Geometry: see drawing. Coordinates: mm, zero at the bounding-box minimum. A direction names the side the tool comes from. Round coordinates to 2 decimals unless told otherwise and drop trailing zeros. Write each loop counter-clockwise with the first axis right and the second up, starting at its lowest first coordinate (ties: lowest second). Pieces come first, ordered by that corner, then holes. Notation, with made-up numbers: M 66,32.5 L 105,32.5 A30 cw 105,56.5 Z; hole C 87.25,40 d7. An arc over 180 degrees is marked long. Use a Markdown table: item, result.
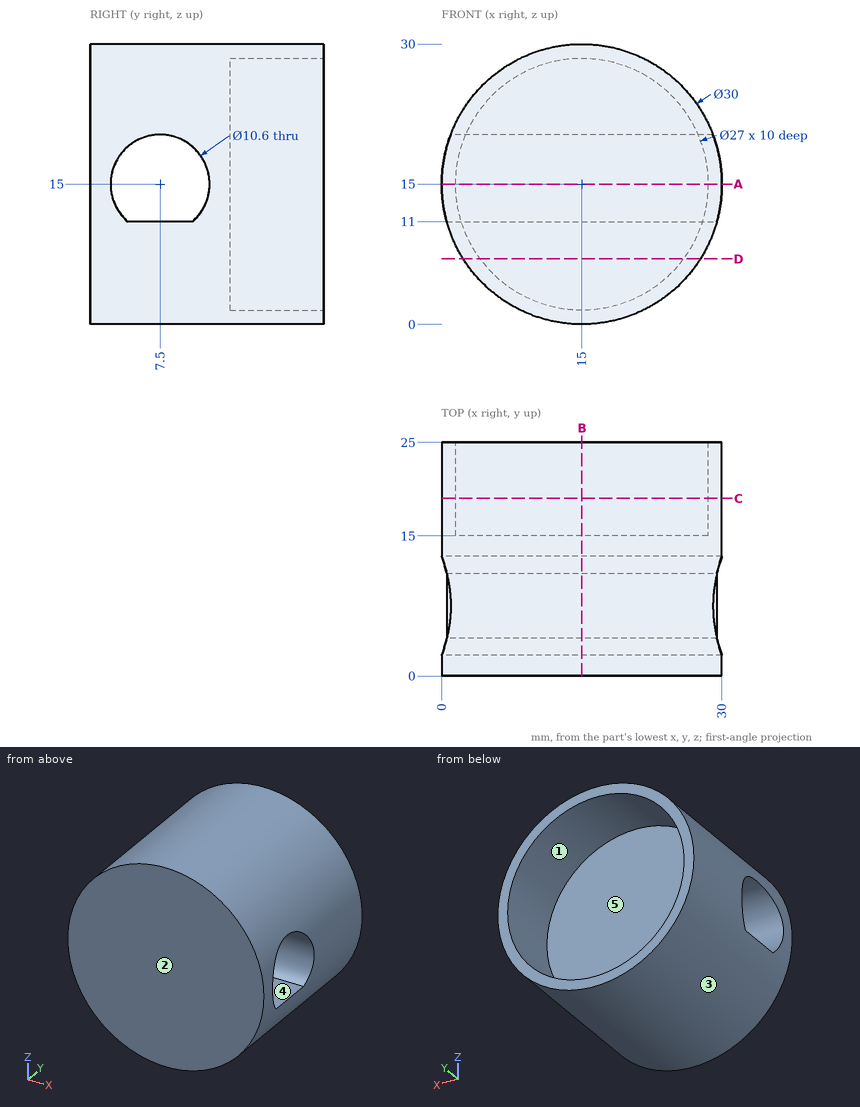
Q1. Section D-D on z = 7. Return loops of the section in (x, y), plus the area to 3 significant figures.
Results are:
| item | result |
|---|---|
| outline | M 2.31,0 L 27.69,0 L 27.69,25 L 25.87,25 L 25.87,15 L 4.13,15 L 4.13,25 L 2.31,25 Z |
| area | 417 mm^2 |
Q2. Reachability of the marked faces 4 and 5 from +Z, -Z, +X, -X, +Y, -Y: full face, straight path, thin tool, end or side. Return the list, or none.
Results are:
| item | result |
|---|---|
| face 4 | +X, -X |
| face 5 | +Y |
Q3. Line query: L1, parallel to Z at x = 15, y = 19.75; L2, parallel to Y at x = 24.5, z = 9; L3, parallel to Z at x = 2.5, y = 7. Output: solid intervals per line, ascending.
Results are:
| item | result |
|---|---|
| L1 | 0 to 1.5, 28.5 to 30 |
| L2 | 0 to 15 |
| L3 | 6.71 to 11, 20.28 to 23.29 |
Q4. First-contact query: pin 1 Ø10 at (y, z) = (12.5, 19) entering from +X; pin 2 Ø10 at (x, y) = (25.5, 21.5) entering from -Z; pin 3 Ø4 at (x, z) = (17, 7.5) entering from +Y; pin 4 Ø12 at (y, z) = (12.5, 3.5) entering from -X. Flat tips, straight axial feed; report the tip coordinate or a pass-through.
Results are:
| item | result |
|---|---|
| pin 1 | x = 30 |
| pin 2 | z = 1.04 |
| pin 3 | y = 15 |
| pin 4 | x = 1.04 |
Q5. Mould query, pull axis X, two halves, no side actions, for the marked faces 1, 2 and 3. Classes: +X half, -X half, draft (parallel to the pull), parting line (faces both ways), or undercut.
Results are:
| item | result |
|---|---|
| face 1 | undercut |
| face 2 | draft |
| face 3 | parting line |
Q6. Section B-B on x = 15. Return loops of the section in (y, z), plus the area to 3 significant figures.
Results are:
| item | result |
|---|---|
| outline | M 0,0 L 25,0 L 25,1.5 L 15,1.5 L 15,28.5 L 25,28.5 L 25,30 L 0,30 Z; hole M 4.02,11 L 10.98,11 A5.3 ccw long Z |
| area | 398 mm^2 |
Q7. Section C-C on y = 19. Return loops of the section in (x, z).
Results are:
| item | result |
|---|---|
| outline | C 15,15 d30; hole C 15,15 d27 |
Q8. Section A-A on z = 15. Return loops of the section in (x, y).
Results are:
| item | result |
|---|---|
| outline | M 0,0 L 30,0 L 30,2.2 L 0,2.2 Z; M 0,12.8 L 30,12.8 L 30,25 L 28.5,25 L 28.5,15 L 1.5,15 L 1.5,25 L 0,25 Z |
